Work out the finished part from the listing and answer in its coordinate system (mm). Face numbers are marked on the shaded views. A direction names the side the tool comes from. Round coordinates to 2 decimals unless told otherwise and drop trailing zeros. Order: outer loops, then holes, each group sorted by start corner. A loop starts at its lowest first (then second) coordinate and runs counter-clockwise, first axis right, second up. Notation, with made-up numbers: (-33, 89) - (17, 89) arc R32 ccw to (17, 116) - close; hole circle Ø10 at (-7.5, -37.5). An arc over 180 degrees is marked (long way). One line per question, with ' | ' between items. Start each with the question number.
from build123d import *

# Parameters (mm, degrees)
F0_R     = 1.5
F1_DEPTH = 15
F2_DEPTH = 12
F3_R     = 1.5
F4_DEPTH = 12


with BuildPart() as f1:
    # F0 (on Front) → F1 (new body)
    with BuildSketch(Plane.XZ):
        with BuildLine():
            Line((0, 11), (0, 15))
            Line((0, 15), (-27.5, 15))
            ThreePointArc((-27.5, 15), (-29.267767, 14.267767), (-30, 12.5))
            Line((-30, 12.5), (-30, -12.5))
            ThreePointArc((-30, -12.5), (-29.267767, -14.267767), (-27.5, -15))
            Line((-27.5, -15), (0, -15))
            Line((0, -15), (0, -11))
            Line((0, -11), (-14, -11))
            ThreePointArc((-14, -11), (-18.242641, -9.242641), (-20, -5))
            Line((-20, -5), (-20, 5))
            ThreePointArc((-20, 5), (-18.242641, 9.242641), (-14, 11))
            Line((-14, 11), (0, 11))
        make_face()
        with Locations((-25, -10)):
            Circle(F0_R, mode=Mode.SUBTRACT)
        with Locations((-25, 10)):
            Circle(F0_R, mode=Mode.SUBTRACT)
        with BuildLine():
            Line((0, -11), (0, 11))
            Line((0, 11), (-14, 11))
            ThreePointArc((-14, 11), (-18.242641, 9.242641), (-20, 5))
            Line((-20, 5), (-20, -5))
            ThreePointArc((-20, -5), (-18.242641, -9.242641), (-14, -11))
            Line((-14, -11), (0, -11))
        make_face()
        with Locations((-10, 0)):
            Circle(F0_R, mode=Mode.SUBTRACT)
        with BuildLine():
            Line((14, 11), (0, 11))
            Line((0, 11), (0, -11))
            Line((0, -11), (14, -11))
            ThreePointArc((14, -11), (18.242641, -9.242641), (20, -5))
            Line((20, -5), (20, 5))
            ThreePointArc((20, 5), (18.242641, 9.242641), (14, 11))
        make_face()
        with Locations((10, 0)):
            Circle(F0_R, mode=Mode.SUBTRACT)
        with BuildLine():
            Line((27.5, 15), (0, 15))
            Line((0, 15), (0, 11))
            Line((0, 11), (14, 11))
            ThreePointArc((14, 11), (18.242641, 9.242641), (20, 5))
            Line((20, 5), (20, -5))
            ThreePointArc((20, -5), (18.242641, -9.242641), (14, -11))
            Line((14, -11), (0, -11))
            Line((0, -11), (0, -15))
            Line((0, -15), (27.5, -15))
            ThreePointArc((27.5, -15), (29.267767, -14.267767), (30, -12.5))
            Line((30, -12.5), (30, 12.5))
            ThreePointArc((30, 12.5), (29.267767, 14.267767), (27.5, 15))
        make_face()
        with Locations((25, -10)):
            Circle(F0_R, mode=Mode.SUBTRACT)
        with Locations((25, 10)):
            Circle(F0_R, mode=Mode.SUBTRACT)
    extrude(amount=F1_DEPTH)

    # F0 (on Front) → F2 (cut)
    with BuildSketch(Plane.XZ):
        with BuildLine():
            Line((0, -11), (0, 11))
            Line((0, 11), (-14, 11))
            ThreePointArc((-14, 11), (-18.242641, 9.242641), (-20, 5))
            Line((-20, 5), (-20, -5))
            ThreePointArc((-20, -5), (-18.242641, -9.242641), (-14, -11))
            Line((-14, -11), (0, -11))
        make_face()
        with Locations((-10, 0)):
            Circle(F0_R, mode=Mode.SUBTRACT)
        with BuildLine():
            Line((14, 11), (0, 11))
            Line((0, 11), (0, -11))
            Line((0, -11), (14, -11))
            ThreePointArc((14, -11), (18.242641, -9.242641), (20, -5))
            Line((20, -5), (20, 5))
            ThreePointArc((20, 5), (18.242641, 9.242641), (14, 11))
        make_face()
        with Locations((10, 0)):
            Circle(F0_R, mode=Mode.SUBTRACT)
    extrude(amount=F2_DEPTH, mode=Mode.SUBTRACT)

    # F3 (on face) → F4 (cut)
    with BuildSketch(Plane.XZ.offset(15)):
        with BuildLine():
            ThreePointArc((30, 12.5), (29.267767, 14.267767), (27.5, 15))
            Line((27.5, 15), (-27.5, 15))
            ThreePointArc((-27.5, 15), (-29.267767, 14.267767), (-30, 12.5))
            Line((-30, 12.5), (-30, -12.5))
            ThreePointArc((-30, -12.5), (-29.267767, -14.267767), (-27.5, -15))
            Line((-27.5, -15), (27.5, -15))
            ThreePointArc((27.5, -15), (29.267767, -14.267767), (30, -12.5))
            Line((30, -12.5), (30, 12.5))
        make_face()
        with Locations((-25, -10)):
            Circle(F3_R, mode=Mode.SUBTRACT)
        with Locations((25, -10)):
            Circle(F3_R, mode=Mode.SUBTRACT)
        with BuildLine():
            ThreePointArc((-21.5, 7.5), (-20.035534, 11.035534), (-16.5, 12.5))
            Line((-16.5, 12.5), (16.5, 12.5))
            ThreePointArc((16.5, 12.5), (20.035534, 11.035534), (21.5, 7.5))
            Line((21.5, 7.5), (21.5, -7.5))
            ThreePointArc((21.5, -7.5), (20.035534, -11.035534), (16.5, -12.5))
            Line((16.5, -12.5), (-16.5, -12.5))
            ThreePointArc((-16.5, -12.5), (-20.035534, -11.035534), (-21.5, -7.5))
            Line((-21.5, -7.5), (-21.5, 7.5))
        make_face(mode=Mode.SUBTRACT)
        with Locations((-25, 10)):
            Circle(F3_R, mode=Mode.SUBTRACT)
        with Locations((25, 10)):
            Circle(F3_R, mode=Mode.SUBTRACT)
    extrude(amount=-F4_DEPTH, mode=Mode.SUBTRACT)


solid = f1.part
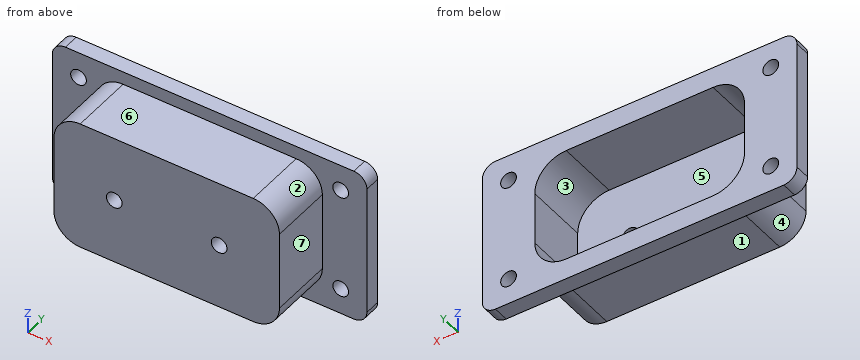
1) Determine the mould class of the marked faces 1, 2 and 3 for opening direction X: released by +X, released by -X, zero draft, split by the parting line, or undercut.
2) Section B-B on y = -5.5 is taken. Give the vertices of the cut face in (x, z).
3) Flat-ended cylindrical pins translate along their axes: pin 1 (1 mm diameter, centred on x = -11, y = -6, fed in from +Z); pin 2 (2.5 mm diameter, centred on x = -25, z = -10, fed in from -Y); pin 3 (3.5 mm diameter, centred on x = -10, z = 0, fed in from -Y); pin 4 (6 mm diameter, centred on y = -10.5, z = -3.5, fed in from +X). Find the tip coordinate at first contact, or state that the pin passes through.
4) Section D-D on x = 25 is taken. Give the vertices of the cut face in (y, z), and give its area (3 significant figures).
5) Straight lines are drawn through the part: line 1 (Z direction, x = -25, y = -2.35); line 2 (Z direction, x = -14, y = -11.25); line 3 (X direction, y = -5, z = -2). For each, find the intervals that lie inside material, in ascending order.
6) Section C-C on z = -3 is taken. Give the vertices of the cut face in (x, y).
7) Section A-A on x = 10 is taken. Give the vertices of the cut face in (y, z), and give its area (3 significant figures).
8) For the marked faces 4, 5, 6 and 7, determine the directions among +Z, -Z, +X, -X, +Y, -Y from which every point of the face is accessible in a straight line to the end or side of a thin tool.
Recorded:
1) face 1: zero draft | face 2: released by +X | face 3: undercut
2) outline: (-21.5, -7.5) arc R5 ccw to (-16.5, -12.5) - (16.5, -12.5) arc R5 ccw to (21.5, -7.5) - (21.5, 7.5) arc R5 ccw to (16.5, 12.5) - (-16.5, 12.5) arc R5 ccw to (-21.5, 7.5) - close; hole (-20, -5) arc R6 ccw to (-14, -11) - (14, -11) arc R6 ccw to (20, -5) - (20, 5) arc R6 ccw to (14, 11) - (-14, 11) arc R6 ccw to (-20, 5) - close
3) pin 1: stops at z = 12.5 | pin 2: passes through | pin 3: stops at y = -15 | pin 4: stops at x = 21.5
4) outline: (-3, -15) - (0, -15) - (0, -11.5) - (-3, -11.5) - close; (-3, -8.5) - (0, -8.5) - (0, 8.5) - (-3, 8.5) - close; (-3, 11.5) - (0, 11.5) - (0, 15) - (-3, 15) - close | area: 72.0 mm²
5) line 1: z = -15 to -11.5, -8.5 to 8.5, 11.5 to 15 | line 2: z = -12.5 to -11, 11 to 12.5 | line 3: x = -21.5 to -20, 20 to 21.5
6) outline: (-30, -3) - (-21.5, -3) - (-21.5, -15) - (21.5, -15) - (21.5, -3) - (30, -3) - (30, 0) - (20, 0) - (20, -12) - (-20, -12) - (-20, 0) - (-30, 0) - close
7) outline: (-15, -12.5) - (-3, -12.5) - (-3, -15) - (0, -15) - (0, -11) - (-12, -11) - (-12, -1.5) - (-15, -1.5) - close; (-15, 1.5) - (-12, 1.5) - (-12, 11) - (0, 11) - (0, 15) - (-3, 15) - (-3, 12.5) - (-15, 12.5) - close | area: 117 mm²
8) face 4: -Z, -X, -Y | face 5: +Y | face 6: +Z, +X, -X, -Y | face 7: +Z, -Z, +X, -Y
